Build history of the part. All positions in model axes, mm. Coordinates: 2 decimals unless noted, no trailing zeros. Loops run counter-clockwise (first coordinate to the right, second up) from the corner with the lowest first, then second, coordinate; pieces in that order, holes last. Notation, with made-up numbers: (60.5, 58.25) - (89.5, 58.25) arc R20 cw to (89.5, 88.25) - close; hole circle Ø11 at (-38.75, -18). An arc over 180 degrees is marked (long way). One line per item, written item: value.
Autodesk Inventor part; units mm, degrees
ref_plane "YZ Plane" through (0, 0, 0) normal (1, 0, 0) x (0, 1, 0)
ref_plane "XZ Plane" through (0, 0, 0) normal (0, 1, 0) x (-1, 0, 0)
ref_plane "XY Plane" through (0, 0, 0) normal (0, 0, 1) x (1, 0, 0)
sketch "Sketch1" plane through (0, 0, 0) normal (0, 0, 1) x (1, 0, 0)
  line L0 (76, 0) -> (76, 180)
  line L1 (0, 180) -> (0, 0)
  line L2 (76, 180) -> (0, 180)
  circle A0 centre (35, 150) radius 10
  line L3 (0, 0) -> (76, 0)
  line L4 (13, 169.7925) -> (13, 8.2181)
  line L5 (63, 169.7925) -> (63, 4.1511)
  circle A1 centre (13, 160) radius 2.1
  circle A2 centre (63, 160) radius 2.1
  circle A3 centre (13, 20) radius 2.1
  circle A4 centre (63, 20) radius 2.1
  point P0 (63, 22.1)
  point P1 (63, 17.9)
  point P2 (13, 22.1)
  point P3 (13, 17.9)
  point P4 (63, 162.1)
  point P5 (63, 157.9)
  point P6 (13, 162.1)
  point P7 (13, 157.9)
  dimension "d1" = 180
  dimension "d26" = 20
  dimension "d27" = 35
  dimension "d28" = 30
  dimension "d29" = 180
  dimension "d30" = 13
  dimension "d31" = 13
  dimension "d32" = 4.2
  dimension "d33" = 4.2
  dimension "d34" = 20
  dimension "d35" = 20
  dimension "d36" = 4.2
  dimension "d37" = 4.2
  dimension "d38" = 20
  dimension "d39" = 20
  dimension "d40" = 76
extrude "Extrusion1" add sketch "Sketch1" along normal blind 3
equation "\"d27\" = 0.5 * d0"
equation "\"d31\" = d30"
equation "\"d33\" = d32"
equation "\"d35\" = d34"
equation "\"d36\" = d33"
equation "\"d37\" = d36"
equation "\"d38\" = d39"
properties part number "BaseC_4" material "PMMA Plastic"
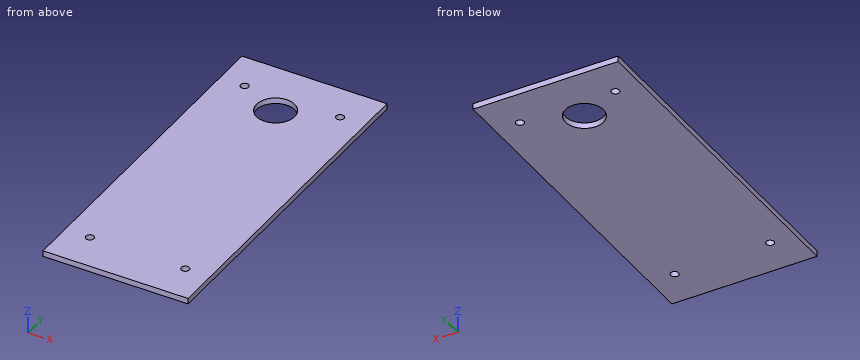
Item 1: Drop a flat-ended pin along its axis: P1, Ø2.5, axis at x = 63, y = 160, coming from the +Z side. Give the stop position or say it passes through.
Check result:
P1: passes through
Item 2: Cut at C-C, the plane y = 150. Write the cut outline in (x, z), then the cut area to 3 significant figures.
Check result:
outline: (0, 0) - (25, 0) - (25, 3) - (0, 3) - close; (45, 0) - (76, 0) - (76, 3) - (45, 3) - close
area: 168 mm^2
Item 3: Cut at D-D, the plane y = 20. Write the cut outline in (x, z).
Check result:
outline: (0, 0) - (10.9, 0) - (10.9, 3) - (0, 3) - close; (15.1, 0) - (60.9, 0) - (60.9, 3) - (15.1, 3) - close; (65.1, 0) - (76, 0) - (76, 3) - (65.1, 3) - close
Item 4: Cut at A-A, the plane x = 63. Write the cut outline in (y, z).
Check result:
outline: (0, 0) - (17.9, 0) - (17.9, 3) - (0, 3) - close; (22.1, 0) - (157.9, 0) - (157.9, 3) - (22.1, 3) - close; (162.1, 0) - (180, 0) - (180, 3) - (162.1, 3) - close
Item 5: Cut at B-B, the plane z = 2.1. Write the cut outline in (x, y), then the cut area to 3 significant figures.
Check result:
outline: (0, 0) - (76, 0) - (76, 180) - (0, 180) - close; hole circle Ø4.2 at (13, 20); hole circle Ø4.2 at (13, 160); hole circle Ø20 at (35, 150); hole circle Ø4.2 at (63, 20); hole circle Ø4.2 at (63, 160)
area: 13,300 mm^2
Item 6: Probe probe 1 along Y at (x, z) = (63, 0.85); probe 2 along X at (y, z) = (20, 1.2); probe 3 along Y at (x, z) = (35, 1.95). List the from-to ranges inside material, lowest first. Write a range as from..to.
Check result:
probe 1: y = 0..17.9, 22.1..157.9, 162.1..180
probe 2: x = 0..10.9, 15.1..60.9, 65.1..76
probe 3: y = 0..140, 160..180
